Autodesk Inventor part; units mm, degrees
ref_plane "YZ Plane" through (0, 0, 0) normal (1, 0, 0) x (0, 1, 0)
ref_plane "XZ Plane" through (0, 0, 0) normal (0, 1, 0) x (-1, 0, 0)
ref_plane "XY Plane" through (0, 0, 0) normal (0, 0, 1) x (1, 0, 0)
sketch "Sketch1" plane through (0, 0, 0) normal (0, 0, 1) x (1, 0, 0)
  line L0 (-29.1905, 5.7934) -> (2.5595, 5.7934) construction
  line L1 (2.5595, 5.7934) -> (2.5595, -6.9066) construction
  line L2 (2.5595, -6.9066) -> (-29.1905, -6.9066) construction
  line L3 (-29.1905, -6.9066) -> (-29.1905, 5.7934) construction
  line L4 (-29.1905, -0.5566) -> (-27.9205, -0.5566) construction
  line L5 (-29.1905, 0.3959) -> (-27.9205, 0.3959)
  line L6 (-29.1905, -1.5091) -> (-27.9205, -1.5091)
  line L7 (-13.3155, 5.7934) -> (-13.3155, -6.9066) construction
  line L8 (2.5595, -0.5566) -> (1.2895, -0.5566) construction
  line L9 (2.5595, 0.3959) -> (1.2895, 0.3959)
  line L10 (2.5595, -1.5091) -> (1.2895, -1.5091)
  line L11 (-14.5855, 5.7934) -> (-12.0455, 5.7934)
  line L12 (-14.5855, -6.9066) -> (-12.0455, -6.9066)
  line L13 (-27.9205, 0.3959) -> (-14.5855, 5.7934)
  line L14 (-12.0455, 5.7934) -> (1.2895, 0.3959)
  line L15 (1.2895, -1.5091) -> (-12.0455, -6.9066)
  line L16 (-14.5855, -6.9066) -> (-27.9205, -1.5091)
  line L17 (-29.1905, 0.3959) -> (-29.1905, -1.5091)
  line L18 (2.5595, -1.5091) -> (2.5595, 0.3959)
  line L19 (0.9577, -0.5566) -> (-12.2417, -5.8992)
  line L20 (-12.2417, -5.8992) -> (-14.3894, -5.8992)
  line L21 (-14.3894, -5.8992) -> (-27.5888, -0.5566)
  line L22 (-27.5888, -0.5566) -> (-14.3894, 4.786)
  line L23 (-14.3894, 4.786) -> (-12.2417, 4.786)
  line L24 (-12.2417, 4.786) -> (0.9577, -0.5566)
  point P0 (0, 0)
  dimension "d0" = 12.7
  dimension "d1" = 31.75
  dimension "d2" = 15.875
  dimension "d3" = 1.905
  dimension "d4" = 2.54
  dimension "d5" = 1.27
extrude "Extrusion1" add sketch "Sketch1" along normal blind 0.254
properties part number "Expanded Metal STOCK"
Model file for the job. Use its own axes, mm. Coordinates: 2 decimals unless noted, no trailing zeros. Order: outer loops, then holes, each group sorted by start corner. A loop starts at its lowest first (then second) coordinate and runs counter-clockwise, first axis right, second up. Notation, with made-up numbers: M 21,26.5 L 31,26.5 A35 cw 31,59.5 Z; hole C 34.5,29.5 d1. An arc over 180 degrees is marked long. Answer as CSV lines item,"result".
(1) Wall check: line 1 along X through (y, z) = (-3.5, 0.1); line 2 along X through (y, z) = (1, 0.15); line 3 along Y through (x, z) = (-20, 0.15). Give the ranges that are in metal, low to high.
Geometry says:
line 1,"x = -23 to -20.32, -6.31 to -3.63"
line 2,"x = -26.43 to -23.74, -2.89 to -0.2"
line 3,"y = -4.72 to -3.63, 2.52 to 3.6"
(2) Band-saw the part on B-B, the plane z = 0.2. List the corners of the cut face in (x, y).
Geometry says:
outline,"M -29.19,-1.51 L -27.92,-1.51 L -14.59,-6.91 L -12.05,-6.91 L 1.29,-1.51 L 2.56,-1.51 L 2.56,0.4 L 1.29,0.4 L -12.05,5.79 L -14.59,5.79 L -27.92,0.4 L -29.19,0.4 Z; hole M -27.59,-0.56 L -14.39,-5.9 L -12.24,-5.9 L 0.96,-0.56 L -12.24,4.79 L -14.39,4.79 Z"
(3) Band-saw the part on C-C, the plane y = -1. List the corners of the cut face in (x, z), then the cut area to 3 significant figures.
Geometry says:
outline,"M -29.19,0 L -26.49,0 L -26.49,0.25 L -29.19,0.25 Z; M -0.14,0 L 2.56,0 L 2.56,0.25 L -0.14,0.25 Z"
area,"1.37 mm2"
(4) Flat gauge pin, fed straight in: pin 1 (6 mm diameter, centred on x = -13.5, y = -0.5, fed in from +Z). Where does the tip first touch, or does it go through?
Geometry says:
pin 1,"passes through"
(5) Band-saw the part on A-A, the plane x = -14. List the corners of the cut face in (y, z), then the cut area to 3 significant figures.
Geometry says:
outline,"M -6.91,0 L -5.9,0 L -5.9,0.25 L -6.91,0.25 Z; M 4.79,0 L 5.79,0 L 5.79,0.25 L 4.79,0.25 Z"
area,"0.512 mm2"
